```python
from build123d import *

# Parameters (mm, degrees)
SKETCH1_R           = 1.75
SKETCH1_R_2         = 1.5
SKETCH1_W           = 20
SKETCH1_H           = 3
SKETCH1_W_2         = 3
SKETCH1_H_2         = 15
SKETCH1_H_3         = 20
BOSS_EXTRUDE1_DEPTH = 5


with BuildPart() as part:
    # Sketch1 → Boss-Extrude1 (new body)
    with BuildSketch(Plane(origin=(0, 0, 0), x_dir=(1, 0, 0), z_dir=(0, 1, 0))):
        Polygon((-151, 147.687817745), (150, 147.687817745), (150, -153.312182255), (-151, -153.312182255), (-151, -133.312182255), (-101.110442892, -79.812182255), (-101.110442892, 74.187817745), (-151, 127.687817745), align=None)
        with Locations(Location((-57.5, 44.187817745, 0), (0, 0, 270))):
            Circle(SKETCH1_R, mode=Mode.SUBTRACT)
        with Locations(Location((-22.5, 44.187817745, 0), (0, 0, 270))):
            Circle(SKETCH1_R, mode=Mode.SUBTRACT)
        with Locations(Location((-22.5, 16.187817745, 0), (0, 0, 270))):
            Circle(SKETCH1_R, mode=Mode.SUBTRACT)
        with Locations(Location((-57.5, 16.187817745, 0), (0, 0, 270))):
            Circle(SKETCH1_R, mode=Mode.SUBTRACT)
        with Locations(Location((107.5, 16.187817745, 0), (0, 0, 90))):
            Circle(SKETCH1_R, mode=Mode.SUBTRACT)
        with Locations(Location((72.5, 16.187817745, 0), (0, 0, 90))):
            Circle(SKETCH1_R, mode=Mode.SUBTRACT)
        with Locations(Location((72.5, 44.187817745, 0), (0, 0, 90))):
            Circle(SKETCH1_R, mode=Mode.SUBTRACT)
        with Locations(Location((107.5, 44.187817745, 0), (0, 0, 90))):
            Circle(SKETCH1_R, mode=Mode.SUBTRACT)
        with Locations(Location((107.5, -49.812182255, 0), (0, 0, 270))):
            Circle(SKETCH1_R, mode=Mode.SUBTRACT)
        with Locations(Location((72.5, -49.812182255, 0), (0, 0, 270))):
            Circle(SKETCH1_R, mode=Mode.SUBTRACT)
        with Locations(Location((72.5, -21.812182255, 0), (0, 0, 270))):
            Circle(SKETCH1_R, mode=Mode.SUBTRACT)
        with Locations(Location((107.5, -21.812182255, 0), (0, 0, 270))):
            Circle(SKETCH1_R, mode=Mode.SUBTRACT)
        with Locations(Location((-57.5, -21.812182255, 0), (0, 0, 90))):
            Circle(SKETCH1_R, mode=Mode.SUBTRACT)
        with Locations(Location((-22.5, -21.812182255, 0), (0, 0, 90))):
            Circle(SKETCH1_R, mode=Mode.SUBTRACT)
        with Locations(Location((-22.5, -49.812182255, 0), (0, 0, 90))):
            Circle(SKETCH1_R, mode=Mode.SUBTRACT)
        with Locations(Location((-57.5, -49.812182255, 0), (0, 0, 90))):
            Circle(SKETCH1_R, mode=Mode.SUBTRACT)
        with Locations(Location((144, -147.312182255, 0), (0, 0, 270))):
            Circle(SKETCH1_R_2, mode=Mode.SUBTRACT)
        with Locations(Location((-145, -147.312182255, 0), (0, 0, 270))):
            Circle(SKETCH1_R_2, mode=Mode.SUBTRACT)
        with Locations(Location((144, 141.687817745, 0), (0, 0, 270))):
            Circle(SKETCH1_R_2, mode=Mode.SUBTRACT)
        with Locations(Location((-145, 141.687817745, 0), (0, 0, 270))):
            Circle(SKETCH1_R_2, mode=Mode.SUBTRACT)
        Polygon((35, 122.5), (35, 92.5), (50, 92.5), (50, 77.187817745), (110, 77.187817745), (110, 74.187817745), (130, 74.187817745), (130, 77.187817745), (127.68177751, 77.187817745), (127.68177751, 92.5), (145, 92.5), (145, 122.5), (130, 122.5), (130, 133.187817745), (50, 133.187817745), (50, 122.5), align=None, mode=Mode.SUBTRACT)
        Polygon((-77.68177751, 77.187817745), (-77.68177751, 92.5), (-95, 92.5), (-95, 122.5), (-80, 122.5), (-80, 133.187817745), (0, 133.187817745), (0, 122.5), (15, 122.5), (15, 92.5), (0, 92.5), (0, 77.187817745), (-60, 77.187817745), (-60, 74.187817745), (-80, 74.187817745), (-80, 77.187817745), align=None, mode=Mode.SUBTRACT)
        Polygon((-60, -82.812182255), (-60, -79.812182255), (-80, -79.812182255), (-80, -82.812182255), (-77.68177751, -82.812182255), (-77.68177751, -98.124364509), (-95, -98.124364509), (-95, -128.124364509), (-80, -128.124364509), (-80, -138.812182255), (0, -138.812182255), (0, -128.124364509), (15, -128.124364509), (15, -98.124364509), (0, -98.124364509), (0, -82.812182255), align=None, mode=Mode.SUBTRACT)
        with Locations((25, -81.312182255)):
            Rectangle(SKETCH1_W, SKETCH1_H, mode=Mode.SUBTRACT)
        Polygon((130, -79.812182255), (130, -82.812182255), (127.68177751, -82.812182255), (127.68177751, -98.124364509), (145, -98.124364509), (145, -128.124364509), (130, -128.124364509), (130, -138.812182255), (50, -138.812182255), (50, -128.124364509), (35, -128.124364509), (35, -98.124364509), (50, -98.124364509), (50, -82.812182255), (110, -82.812182255), (110, -79.812182255), align=None, mode=Mode.SUBTRACT)
        with Locations((25, 75.687817745)):
            Rectangle(SKETCH1_W, SKETCH1_H, mode=Mode.SUBTRACT)
        with Locations((-3.5, 22.187817745)):
            Rectangle(SKETCH1_W_2, SKETCH1_H_2, mode=Mode.SUBTRACT)
        with Locations((-3.5, -27.812182255)):
            Rectangle(SKETCH1_W_2, SKETCH1_H_2, mode=Mode.SUBTRACT)
        with Locations((53.5, -27.812182255)):
            Rectangle(SKETCH1_W_2, SKETCH1_H_2, mode=Mode.SUBTRACT)
        with Locations((53.5, 22.187817745)):
            Rectangle(SKETCH1_W_2, SKETCH1_H_2, mode=Mode.SUBTRACT)
        with Locations((146.5, 64.187817745)):
            Rectangle(SKETCH1_W_2, SKETCH1_H_3, mode=Mode.SUBTRACT)
        with Locations((146.5, -0.812182255)):
            Rectangle(SKETCH1_W_2, SKETCH1_H_3, mode=Mode.SUBTRACT)
        with Locations((146.5, -65.812182255)):
            Rectangle(SKETCH1_W_2, SKETCH1_H_3, mode=Mode.SUBTRACT)
    extrude(amount=BOSS_EXTRUDE1_DEPTH)


solid = part.part
```
Here's how the part is built. I have some questions about the finished solid (model axes, mm). A direction names the side the tool comes from. Give positions to 0.01 mm unless a question says otherwise; leave off trailing zeros. Loops run counter-clockwise (first coordinate to the right, second up) from the corner with the lowest first, then second, coordinate; pieces in that order, holes last. Notation, with made-up numbers: (51, 78.5) -> (64, 78.5) arc R36 ccw to (64, 112.5) -> close; hole circle Ø9 at (-2, 21.25). An arc over 180 degrees is marked (long way). Use one line per item in the form item = value. Start each with the question number.
1) Imagine slicing it at D-D (z = -50.5). Please give me the cut outline in (x, y), then the cut area to 3 significant figures.
2) Imagine slicing it at A-A (x = 41.5). Please give me the cut outline in (y, z).
3) Thinking about a two-plate mould opening in Z: for faces 3 (the face through (-125.706, 2.465, -100.563)), 4 (the face through (2, 0, 1)), which applies, +Z half, -Z half, draft (parallel to the pull), parting line (faces both ways), or undercut?
4) Which directions (+Z, -Z, +X, -X, +Y, -Y) give clear straight access to the entire face, cutting with the end or side of a thin tool? Please do faces 1 (the face through (-126.404, 2.465, 106.937)), 2 (the face through (2, 5, 1)).
5) Please list where these lines run through material, in increasing order: line 1 along X through (y, z) = (3.9, -18); line 2 along Z through (x, y) = (-54, 4.7); line 3 along Z through (x, y) = (-94, 4.4).
6) For P1, Ø2.5, axis at y = 1.5, z = -75, coming from the -X side; P2, Ø1.5, axis at y = 2.5, z = 64, coming from the -X side; P3, Ø3, axis at x = -57.5, z = 21.81, coming from the -Y side, each with a flat end and sliding along its axis, tell me the tip position at first contact or that it passes through.
7) Imagine slicing it at C-C (y = 3.4). Count the separate pieces of the cut face and the enclosed holes in it, then the cut area to 3 significant figures.
8) Imagine slicing it at B-B (x = -30). Please give me the cut outline in (y, z), then the cut area to 3 significant figures.
Check values:
q1.outline = (-101.11, 0) -> (150, 0) -> (150, 5) -> (-101.11, 5) -> close
q1.area = 1,260 mm^2
q2.outline = (0, -147.69) -> (5, -147.69) -> (5, -122.5) -> (0, -122.5) -> close; (0, -92.5) -> (5, -92.5) -> (5, 98.12) -> (0, 98.12) -> close; (0, 128.12) -> (5, 128.12) -> (5, 153.31) -> (0, 153.31) -> close
q3.face_3 = undercut
q3.face_4 = draft
q4.face_1 = -X, +Y, -Y
q4.face_2 = +Z, -Z, +X, -X, +Y
q5.line_1 = -101.11 to -5, -2 to 52, 55 to 150
q5.line_2 = -147.69 to -133.19, -77.19 to 82.81, 138.81 to 153.31
q5.line_3 = -147.69 to -122.5, -92.5 to 98.12, 128.12 to 153.31
q6.P1 = -103.03
q6.P2 = -101.11
q6.P3 = through
q7.separate_pieces = 1
q7.enclosed_holes = 33
q7.area = 58,000 mm^2
q8.outline = (0, -147.69) -> (5, -147.69) -> (5, -133.19) -> (0, -133.19) -> close; (0, -77.19) -> (5, -77.19) -> (5, 82.81) -> (0, 82.81) -> close; (0, 138.81) -> (5, 138.81) -> (5, 153.31) -> (0, 153.31) -> close
q8.area = 945 mm^2
